```python
from build123d import *

# Parameters (mm, degrees)
SKETCH_1_W          = 130
SKETCH_1_H          = 68
EXTRUDE_1_DEPTH     = 3
SKETCH_2_R          = 1.7
CUT_EXTRUDE_1_DEPTH = 74.416619372
SKETCH_3_R          = 1.5
CUT_EXTRUDE_2_DEPTH = 74.416619372
SKETCH_4_W          = 27
SKETCH_4_H          = 56
SKETCH_4_W_2        = 24
SKETCH_4_H_2        = 24
CUT_EXTRUDE_3_DEPTH = 74.416619372
EXTRUDE_1_2_DEPTH   = 3
EXTRUDE_START       = -3
EXTRUDE_3_DEPTH     = 3
FILLET_2_R          = 1
FILLET_3_R          = 1.6


# Read off the part's stored shape, not the designer's step: 拉伸-薄壁3
with BuildPart() as part:
    # 草图1 → Extrude 1 (new body)
    with BuildSketch(Plane.XY):
        Rectangle(SKETCH_1_W, SKETCH_1_H)
    extrude(amount=EXTRUDE_1_DEPTH)

    # 草图2 → 切除-拉伸1 (cut, through all)
    with BuildSketch(Plane.XY.offset(3)):
        with Locations((-57, -29)):
            Circle(SKETCH_2_R)
        with Locations((-57, -19)):
            Circle(SKETCH_2_R)
        with Locations((-57, 19)):
            Circle(SKETCH_2_R)
        with Locations((-57, 29)):
            Circle(SKETCH_2_R)
        with Locations(Location((57, 29, 0), (0, 0, 180))):
            Circle(SKETCH_2_R)
        with Locations(Location((57, 19, 0), (0, 0, 180))):
            Circle(SKETCH_2_R)
        with Locations(Location((57, -19, 0), (0, 0, 180))):
            Circle(SKETCH_2_R)
        with Locations(Location((57, -29, 0), (0, 0, 180))):
            Circle(SKETCH_2_R)
    extrude(amount=-CUT_EXTRUDE_1_DEPTH, mode=Mode.SUBTRACT)

    # 草图3 → 切除-拉伸2 (cut, through all)
    with BuildSketch(Plane.XY.offset(3)):
        with Locations((-18, 18)):
            Circle(SKETCH_3_R)
        with Locations((18, 18)):
            Circle(SKETCH_3_R)
        with Locations((18, -18)):
            Circle(SKETCH_3_R)
        with Locations((-18, -18)):
            Circle(SKETCH_3_R)
    extrude(amount=-CUT_EXTRUDE_2_DEPTH, mode=Mode.SUBTRACT)

    # 草图4 → 切除-拉伸3 (cut, through all)
    with BuildSketch(Plane.XY.offset(3)):
        with Locations((-37.5, 0)):
            Rectangle(SKETCH_4_W, SKETCH_4_H)
        Rectangle(SKETCH_4_W_2, SKETCH_4_H_2)
        with Locations((37.5, 0)):
            Rectangle(SKETCH_4_W, SKETCH_4_H)
        Polygon((-17.5, 28), (-12, 18), (12, 18), (17.5, 28), align=None)
        Polygon((12, -18), (17.5, -28), (-17.5, -28), (-12, -18), align=None)
    extrude(amount=-CUT_EXTRUDE_3_DEPTH, mode=Mode.SUBTRACT)

    # 草图5 → Extrude 1 2 (add, through all)
    with BuildSketch(Plane.XY.offset(3)):
        Polygon((-13.237436867, 10.762563133), (10.762563133, -13.237436867), (13.237436867, -10.762563133), (-10.762563133, 13.237436867), align=None)
        Polygon((-10.762563133, -13.237436867), (13.237436867, 10.762563133), (10.762563133, 13.237436867), (-13.237436867, -10.762563133), align=None)
        Polygon((-10.879677301, 16.655612761), (0, 25.722010511), (10.879677301, 16.655612761), (13.120322699, 19.344387239), (0, 30.277989489), (-13.120322699, 19.344387239), align=None)
        Polygon((-13.120322699, -19.344387239), (0, -30.277989489), (13.120322699, -19.344387239), (10.879677301, -16.655612761), (0, -25.722010511), (-10.879677301, -16.655612761), align=None)
    extrude(amount=-EXTRUDE_1_2_DEPTH)

    # 拉伸-薄壁3 outline → 拉伸-薄壁3 (add)
    with BuildSketch(Plane.XY.offset(3).offset(EXTRUDE_START)):
        Polygon((51, -23.678077702), (31.060425073, -3), (51, -3), (51, 3), (31.060425073, 3), (51, 23.678077702), (51, 28), (46.83243207, 28), (24, 4.321922298), (24, -4.321922298), (46.83243207, -28), (51, -28), align=None)
        Polygon((-51, 23.678077702), (-31.060425073, 3), (-51, 3), (-51, -3), (-31.060425073, -3), (-51, -23.678077702), (-51, -28), (-46.83243207, -28), (-24, -4.321922298), (-24, 4.321922298), (-46.83243207, 28), (-51, 28), align=None)
    extrude(amount=EXTRUDE_3_DEPTH)

    # 圆角2
    fillet_2_edges = [part.edges().sort_by_distance(p)[0] for p in [
        (65, -34, 1.5),
        (-65, -34, 1.5),
        (-65, 34, 1.5),
        (65, 34, 1.5),
    ]]
    fillet(fillet_2_edges, radius=FILLET_2_R)

    # 圆角3
    fillet_3_edges = [part.edges().sort_by_distance(p)[0] for p in [
        (-24, 28, 1.5),
        (-24, -28, 1.5),
        (17.5, -28, 1.5),
        (-17.5, -28, 1.5),
        (-17.5, 28, 1.5),
        (17.5, 28, 1.5),
        (24, -28, 1.5),
        (24, 28, 1.5),
        (9.525126266, 12, 1.5),
        (-9.525126266, 12, 1.5),
        (-12, -9.525126266, 1.5),
        (-12, 9.525126266, 1.5),
        (-9.525126266, -12, 1.5),
        (9.525126266, -12, 1.5),
        (12, 9.525126266, 1.5),
        (12, -9.525126266, 1.5),
        (2.474873734, 0, 1.5),
        (0, -2.474873734, 1.5),
        (-2.474873734, 0, 1.5),
        (0, 2.474873734, 1.5),
        (-12.859127464, 19.562049935, 1.5),
        (-9.266412613, 18, 1.5),
        (9.266412613, 18, 1.5),
        (12.859127464, 19.562049935, 1.5),
        (2.733587387, 28, 1.5),
        (0, 25.722010511, 1.5),
        (-2.733587387, 28, 1.5),
        (-12.859127464, -19.562049935, 1.5),
        (2.733587387, -28, 1.5),
        (9.266412613, -18, 1.5),
        (-9.266412613, -18, 1.5),
        (0, -25.722010511, 1.5),
        (12.859127464, -19.562049935, 1.5),
        (-2.733587387, -28, 1.5),
        (46.83243207, 28, 1.5),
        (24, -4.321922298, 1.5),
        (51, 23.678077702, 1.5),
        (51, -23.678077702, 1.5),
        (31.060425073, -3, 1.5),
        (31.060425073, 3, 1.5),
        (46.83243207, -28, 1.5),
        (24, 4.321922298, 1.5),
        (51, 3, 1.5),
        (51, -3, 1.5),
        (-46.83243207, -28, 1.5),
        (-24, 4.321922298, 1.5),
        (-51, -23.678077702, 1.5),
        (-51, 23.678077702, 1.5),
        (-46.83243207, 28, 1.5),
        (-24, -4.321922298, 1.5),
        (-31.060425073, -3, 1.5),
        (-51, -3, 1.5),
        (-31.060425073, 3, 1.5),
        (-51, 3, 1.5),
    ]]
    fillet(fillet_3_edges, radius=FILLET_3_R)


solid = part.part
```
The model under review builds one solid part; all positions refer to its coordinate system, in mm. Round coordinates to 2 decimals unless told otherwise and drop trailing zeros. Loops run counter-clockwise (first coordinate to the right, second up) from the corner with the lowest first, then second, coordinate; pieces in that order, holes last. Notation, with made-up numbers: (-18, 16) -> (-2, 16) arc R29 cw to (-2, 45) -> close; hole circle Ø1 at (29, 50.5). An arc over 180 degrees is marked (long way). Answer in a Markdown table with one row per item.
1) Draft analysis for pull direction X (two halves, no side actions). For faces 1 (the flat face through (3.923, -6.398, 1.521)), 2 (the flat face through (-1, -34, 1)), state which applies: pulls with the +X half, pulls with the -X half, needs draft (parallel to the pull), parting line crosses it, or undercut.
Taken from the geometry:
| item | result |
|---|---|
| face 1 | undercut |
| face 2 | needs draft |
2) Consider section A-A, the plane x = -57. Write out the cut boundary in (y, z), plus the area to 3 significant figures.
Taken from the geometry:
| item | result |
|---|---|
| outline | (-34, 0) -> (-30.7, 0) -> (-30.7, 3) -> (-34, 3) -> close; (-27.3, 0) -> (-20.7, 0) -> (-20.7, 3) -> (-27.3, 3) -> close; (-17.3, 0) -> (17.3, 0) -> (17.3, 3) -> (-17.3, 3) -> close; (20.7, 0) -> (27.3, 0) -> (27.3, 3) -> (20.7, 3) -> close; (30.7, 0) -> (34, 0) -> (34, 3) -> (30.7, 3) -> close |
| area | 163 mm² |
3) Consider section D-D, the plane z = 0.5. Count the separate pieces of the cut face and the enclosed holes in it, plus the area to 3 significant figures.
Taken from the geometry:
| item | result |
|---|---|
| separate pieces | 1 |
| enclosed holes | 30 |
| area | 6,200 mm² |
4) Consider section B-B, the plane x = 18. Write out the cut boundary in (y, z), plus the area to 3 significant figures.
Taken from the geometry:
| item | result |
|---|---|
| outline | (-34, 0) -> (-19.5, 0) -> (-19.5, 3) -> (-34, 3) -> close; (-16.5, 0) -> (16.5, 0) -> (16.5, 3) -> (-16.5, 3) -> close; (19.5, 0) -> (34, 0) -> (34, 3) -> (19.5, 3) -> close |
| area | 186 mm² |
5) Wall thickness on line 1 along Y through (x, z) = (57, 1.6); line 2 along Y through (x, z) = (-18, 1.9); line 3 along Y through (x, z) = (13.5, 0.65): over which ranges is each line inside the solid? List them lowest first.
Taken from the geometry:
| item | result |
|---|---|
| line 1 | y = -34 to -30.7, -27.3 to -20.7, -17.3 to 17.3, 20.7 to 27.3, 30.7 to 34 |
| line 2 | y = -34 to -19.5, -16.5 to 16.5, 19.5 to 34 |
| line 3 | y = -34 to -28, -20.88 to 20.88, 28 to 34 |
6) For pin 1 Ø5 at (x, y) = (-46.5, 9) entering from -Z, flat-tipped, find the tip position at first contact; note if it passes through.
Taken from the geometry:
| item | result |
|---|---|
| pin 1 | passes through |
7) Consider section C-C, the plane y = 15. Write out the cut boundary in (x, z), plus the area to 3 significant figures.
Taken from the geometry:
| item | result |
|---|---|
| outline | (-65, 0) -> (-51, 0) -> (-51, 3) -> (-65, 3) -> close; (-42.63, 0) -> (-34.3, 0) -> (-34.3, 3) -> (-42.63, 3) -> close; (-24, 0) -> (24, 0) -> (24, 3) -> (-24, 3) -> close; (34.3, 0) -> (42.63, 0) -> (42.63, 3) -> (34.3, 3) -> close; (51, 0) -> (65, 0) -> (65, 3) -> (51, 3) -> close |
| area | 278 mm² |
